The figure shows three views and two pictorial views of one solid part (mm, origin at its lowest corner). Answer the questions. Round coordinates to 2 decimals unless told otherwise and drop trailing zeros. Order: outer loops, then holes, each group sorted by start corner. A loop starts at its lowest first (then second) coordinate and runs counter-clockwise, first axis right, second up. Notation, with made-up numbers: (16, -32) - (69, -32) arc R16 ccw to (69, -24) - close; hole circle Ø9 at (81.5, -17.75). An arc over 180 degrees is marked (long way). Use CSV: the item, a comma, the result in double quotes. Start each with the question number.
Item 1: A straight line is drawn through the part: line 1 along X through (y, z) = (0.7, 25.75). Find the intervals that lie inside material, in ascending order. Write a range as [from, to].
Item 2: Find section B-B, the plane z = 2.5. Give the vertices of the cut face in (x, y).
Item 3: Find section A-A, the plane y = 1.45. Give the vertices of the cut face in (x, z).
Item 4: Flat-ended cylindrical pins translate along their axes: P1, Ø1.5, axis at x = 3, y = 2.5, coming from the +Z side; P2, Ø1.5, axis at y = 3.5, z = 3.5, coming from the +X side; P3, Ø1.5, axis at y = 1.5, z = 2.5, coming from the -X side. Find the tip coordinate at first contact, or state that the pin passes through.
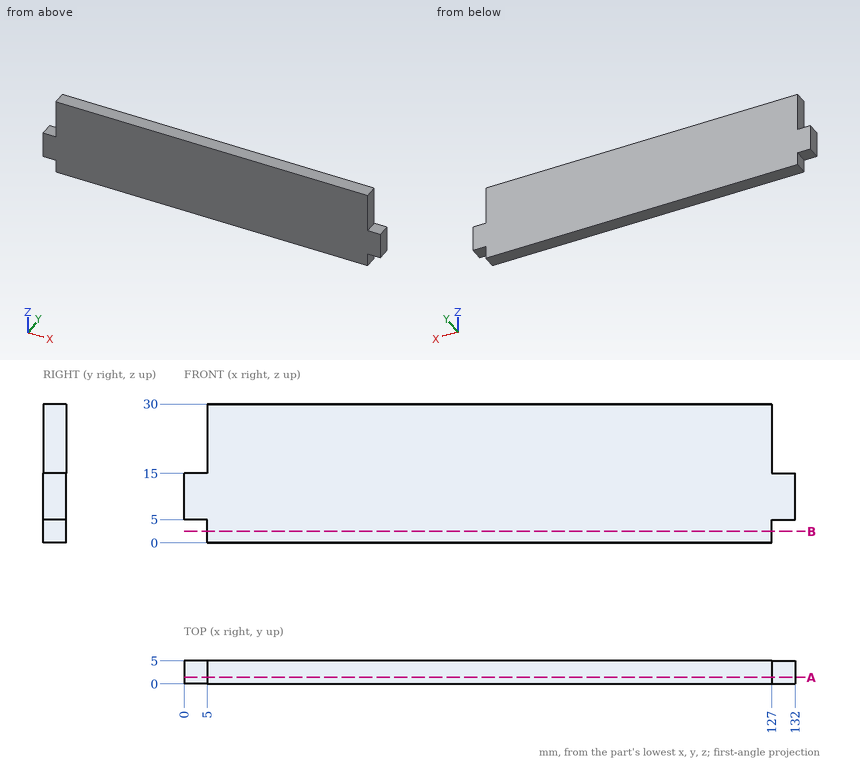
Worked out:
1,line 1,"x = [5, 127]"
2,outline,"(5, 0) - (127, 0) - (127, 5) - (5, 5) - close"
3,outline,"(0, 5) - (5, 5) - (5, 0) - (127, 0) - (127, 5) - (132, 5) - (132, 15) - (127, 15) - (127, 30) - (5, 30) - (5, 15) - (0, 15) - close"
4,P1,"stops at z = 15"
4,P2,"stops at x = 127"
4,P3,"stops at x = 5"
